Geometry: final body of the model. Coordinates: model frame, mm. A direction names the side the tool comes from. Give positions to 0.01 mm unless a question says otherwise; leave off trailing zeros. Order: outer loops, then holes, each group sorted by start corner. A loop starts at its lowest first (then second) coordinate and runs counter-clockwise, first axis right, second up. Notation, with made-up numbers: (86, 43.5) -> (114, 43.5) arc R22 ccw to (114, 68.5) -> close; hole circle Ø5 at (20.25, -31). An arc over 180 degrees is marked (long way). One line per item, written item: value. Start each with the question number.
```python
from build123d import *
from build123d.topology import SkipClean

# Parameters (mm, degrees)
BOSS_EXTRUDE1_DEPTH = 21
SKETCH2_R           = 12
CUT_EXTRUDE1_DEPTH  = 21
SKETCH3_R           = 26
CUT_EXTRUDE2_DEPTH  = 273.603191471
SKETCH5_R           = 31.5
SKETCH5_R_2         = 26
BOSS_EXTRUDE2_DEPTH = 35
SKETCH4_R           = 5
BOSS_EXTRUDE3_DEPTH = 7
CUT_EXTRUDE3_DEPTH  = 20
CUT_EXTRUDE5_REACH  = 280.977
CUT_EXTRUDE6_REACH  = 280.977
CUT_EXTRUDE7_START  = -2.5
CUT_EXTRUDE7_DEPTH  = 274.030851267


with BuildPart() as part:
    # Sketch1 → Boss-Extrude1 (new, symmetric)
    with BuildSketch(Plane(origin=(0, 0, 0), x_dir=(1, 0, 0), z_dir=(0, 1, 0))):
        with BuildLine():
            Line((60.430871603, 12.898377286), (220, 8.719912605))
            ThreePointArc((220, 8.719912605), (230.604685788, 10.075596562), (240.30539773, 14.569306326))
            ThreePointArc((240.30539773, 14.569306326), (267.5, 0), (240.30539773, -14.569306326))
            ThreePointArc((240.30539773, -14.569306326), (230.604685788, -10.075596562), (220, -8.719912605))
            Line((220, -8.719912605), (60.430871603, -12.898377286))
            ThreePointArc((60.430871603, -12.898377286), (37.890504435, -16.634432055), (17.222812986, -26.374698346))
            ThreePointArc((17.222812986, -26.374698346), (-31.5, 0), (17.222812986, 26.374698346))
            ThreePointArc((17.222812986, 26.374698346), (37.890504435, 16.634432055), (60.430871603, 12.898377286))
        make_face()
    extrude(amount=BOSS_EXTRUDE1_DEPTH, both=True)

    # Sketch2 → Cut-Extrude1 (cut, symmetric)
    with BuildSketch(Plane(origin=(0, 0, 0), x_dir=(1, 0, 0), z_dir=(0, 1, 0))):
        with Locations(Location((250, 0, 0), (0, 0, 270))):
            Circle(SKETCH2_R)
    extrude(amount=CUT_EXTRUDE1_DEPTH, both=True, mode=Mode.SUBTRACT)

    # Sketch3 → Cut-Extrude2 (cut, through all)
    with BuildSketch(Plane.XZ.offset(21)):
        with Locations(Location((0, 0, 0), (0, 0, 270))):
            Circle(SKETCH3_R)
    extrude(amount=-CUT_EXTRUDE2_DEPTH, mode=Mode.SUBTRACT)

    # Sketch5 → Boss-Extrude2 (add, symmetric)
    with SkipClean():  # the faces are left unmerged after this step: merging them gives an invalid solid
        with BuildSketch(Plane(origin=(0, 0, 0), x_dir=(1, 0, 0), z_dir=(0, 1, 0))):
            with Locations(Location((0, 0, 0), (0, 0, 270))):
                Circle(SKETCH5_R)
            with Locations(Location((0, 0, 0), (0, 0, 90))):
                Circle(SKETCH5_R_2, mode=Mode.SUBTRACT)
        extrude(amount=BOSS_EXTRUDE2_DEPTH, both=True)

    # Sketch4 → Boss-Extrude3 (add)
    with BuildSketch(Plane.XZ.offset(21)):
        with BuildLine():
            Line((87.482015231, 12.190018161), (87.482015231, -12.190018161))
            ThreePointArc((87.482015231, -12.190018161), (51.997088566, -22.622612499), (26.373739078, -49.29587638))
            ThreePointArc((26.373739078, -49.29587638), (17.709961948, -55.714405462), (7.181946677, -53.386435492))
            ThreePointArc((7.181946677, -53.386435492), (-14.855989459, -42.122318837), (-39.406288617, -38.986435492))
            ThreePointArc((-39.406288617, -38.986435492), (-50.326951915, -33.896458963), (-52.376901133, -22.023529412))
            ThreePointArc((-52.376901133, -22.023529412), (-48.925892025, 0), (-52.376901133, 22.023529412))
            ThreePointArc((-52.376901133, 22.023529412), (-50.326951915, 33.896458963), (-39.406288617, 38.986435492))
            ThreePointArc((-39.406288617, 38.986435492), (-14.855989459, 42.122318837), (7.181946677, 53.386435492))
            ThreePointArc((7.181946677, 53.386435492), (17.709961948, 55.714405462), (26.373739078, 49.29587638))
            ThreePointArc((26.373739078, 49.29587638), (51.997088566, 22.622612499), (87.482015231, 12.190018161))
        make_face()
        with Locations(Location((15, 43, 0), (0, 0, 270))):
            Circle(SKETCH4_R, mode=Mode.SUBTRACT)
        with Locations(Location((-40, 26, 0), (0, 0, 270))):
            Circle(SKETCH4_R, mode=Mode.SUBTRACT)
        with Locations(Location((15, -43, 0), (0, 0, 90))):
            Circle(SKETCH4_R, mode=Mode.SUBTRACT)
        with Locations(Location((-40, -26, 0), (0, 0, 90))):
            Circle(SKETCH4_R, mode=Mode.SUBTRACT)
    boss_extrude3 = extrude(amount=-BOSS_EXTRUDE3_DEPTH)

    # Mirror1: Boss-Extrude3 across plane
    add(boss_extrude3.mirror(Plane.ZX))

    # Sketch6 → Cut-Extrude3 (cut, symmetric)
    with BuildSketch(Plane.XY):
        with BuildLine():
            Line((123.875759549, 11.370189358), (232.5, 9))
            Line((232.5, 9), (232.5, 21))
            Line((232.5, 21), (88, 21))
            ThreePointArc((88, 21), (105.356268471, 14.018307807), (123.875759549, 11.370189358))
        make_face()
    cut_extrude3 = extrude(amount=CUT_EXTRUDE3_DEPTH, both=True, mode=Mode.SUBTRACT)

    # Mirror2: Cut-Extrude3 across plane
    add(cut_extrude3.mirror(Plane.ZX), mode=Mode.SUBTRACT)

    # Cut-Extrude5: up to this face of the body (flat: up to its plane)
    cut_extrude5_end = Plane(part.part.faces().sort_by_distance((176.036341328, 10.232041415, 0))[0])
    # Sketch7 → Cut-Extrude5 (cut, up to the picked face)
    with BuildSketch(Plane(origin=(0, 21, 0), x_dir=(1, 0, 0), z_dir=(0, 1, 0)), mode=Mode.PRIVATE) as cut_extrude5_sk1:
        with BuildLine():
            Line((232.5, 10.680424072), (232.5, 0))
            ThreePointArc((232.5, 0), (234.574282193, 8.264213825), (240.30539773, 14.569306326))
            ThreePointArc((240.30539773, 14.569306326), (236.524290746, 12.380817442), (232.5, 10.680424072))
        make_face()
    cut_extrude5_tool1 = split(extrude(cut_extrude5_sk1.sketch, amount=-CUT_EXTRUDE5_REACH, mode=Mode.PRIVATE), bisect_by=cut_extrude5_end, keep=Keep.BOTH, mode=Mode.PRIVATE)
    cut_extrude5 = cut_extrude5_tool1.solids().sort_by(Axis((234.203382, 21, -9.039339), (0, -1, 0)))[0]
    add(cut_extrude5, mode=Mode.SUBTRACT)

    # Mirror10: Cut-Extrude5 across plane
    with SkipClean():  # the faces are left unmerged after this step: merging them gives an invalid solid
        add(cut_extrude5.mirror(Plane.XY), mode=Mode.SUBTRACT)

    # Cut-Extrude6: up to this face of the body (flat: up to its plane)
    cut_extrude6_end = Plane(part.part.faces().sort_by_distance((176.036341328, -10.232041415, 0))[0])
    # Sketch9 → Cut-Extrude6 (cut, up to the picked face)
    with BuildSketch(Plane.XZ.offset(21), mode=Mode.PRIVATE) as cut_extrude6_sk1:
        with BuildLine():
            Line((232.5, 10.680424072), (232.5, 0))
            ThreePointArc((232.5, 0), (234.574282193, 8.264213825), (240.30539773, 14.569306326))
            ThreePointArc((240.30539773, 14.569306326), (236.524290746, 12.380817442), (232.5, 10.680424072))
        make_face()
    cut_extrude6_tool1 = split(extrude(cut_extrude6_sk1.sketch, amount=-CUT_EXTRUDE6_REACH, mode=Mode.PRIVATE), bisect_by=cut_extrude6_end, keep=Keep.BOTH, mode=Mode.PRIVATE)
    # Sketch9 → Cut-Extrude6 (cut, up to the picked face)
    with BuildSketch(Plane.XZ.offset(21), mode=Mode.PRIVATE) as cut_extrude6_sk2:
        with BuildLine():
            Line((232.5, 0), (232.5, -10.680424072))
            ThreePointArc((232.5, -10.680424072), (236.524290746, -12.380817442), (240.30539773, -14.569306326))
            ThreePointArc((240.30539773, -14.569306326), (234.574282193, -8.264213825), (232.5, 0))
        make_face()
    cut_extrude6_tool2 = split(extrude(cut_extrude6_sk2.sketch, amount=-CUT_EXTRUDE6_REACH, mode=Mode.PRIVATE), bisect_by=cut_extrude6_end, keep=Keep.BOTH, mode=Mode.PRIVATE)
    add(cut_extrude6_tool1.solids().sort_by(Axis((234.203382, -21, 9.039339), (0, 1, 0)))[0], mode=Mode.SUBTRACT)
    add(cut_extrude6_tool2.solids().sort_by(Axis((234.203382, -21, -9.039339), (0, 1, 0)))[0], mode=Mode.SUBTRACT)

    # Sketch10 → Cut-Extrude7 (cut, through all)
    with SkipClean():  # the faces are left unmerged after this step: merging them gives an invalid solid
        with BuildSketch(Plane(origin=(0, 0, 0), x_dir=(1, 0, 0), z_dir=(0, 1, 0)).offset(CUT_EXTRUDE7_START)):
            with BuildLine():
                Line((220, -6), (70, -6))
                ThreePointArc((70, -6), (64, 0), (70, 6))
                Line((70, 6), (220, 6))
                ThreePointArc((220, 6), (226, 0), (220, -6))
            make_face()
        cut_extrude7 = extrude(amount=-CUT_EXTRUDE7_DEPTH, mode=Mode.SUBTRACT)

    # Mirror11: Cut-Extrude7 across plane
    with SkipClean():  # the faces are left unmerged after this step: merging them gives an invalid solid
        add(cut_extrude7.mirror(Plane.ZX), mode=Mode.SUBTRACT)


solid = part.part
```
1. Cut plane B-B, the plane x = 250. Return loops of the section in (y, z).
2. Cut plane A-A, the plane y = -17. Return loops of the section in (x, z).
3. Draft query along X for faces 5 (the flat face through (0, 21, 0)), 6 (the cylindrical face through (-31.486, 0.196, 0.948)), 7 (the flat face through (26, -35, 5)). Return one class per face: pulls with the +X half, pulls with the -X half, needs draft (parallel to the pull), parting line crosses it, or undercut.
4. Access query for faces 1 (the cylindrical face through (105.103, 14.087, -9.045)), 2 (the flat face through (34, -21, -1)), 3 (the cylindrical face through (51.55, 17.549, 22.896)), 4 (the flat face through (34, 21, -1)). Directions: +Z, -Z, +X, -X, +Y, -Y. A direction counts if a zero-diameter tool reaches every point of the face in a straight line with its end or side. Return the directions, or none.
5. Pin query (flat end, axial travel): P1, Ø9, axis at x = 125, y = -14.5, coming from the +Z side; P2, Ø12, axis at x = 151.5, y = -16.5, coming from the -Z side; P3, Ø15, axis at x = 161.5, y = 15, coming from the -Z side. Return the tip coordinate at first contact, or that it passes through.
6. Cut plane C-C, the plane z = 43. Return loops of the section in (x, y).
7. Material intervals for L1, parallel to Z at x = 0, y = -32; L2, parallel to X at y = 11, z = 1, sorted ascending. Write a range as [from, to].
8. Cut plane D-D, the plane x = 183. Return loops of the section in (y, z), then the cut area to 3 significant figures.
Answers follow:
1. outline: (-21, -17.5) -> (21, -17.5) -> (21, -12) -> (-21, -12) -> close; (-21, 12) -> (21, 12) -> (21, 17.5) -> (-21, 17.5) -> close
2. outline: (-52.38, -22.02) arc R13 ccw to (-39.41, -38.99) arc R72 cw to (7.18, -53.39) arc R13 ccw to (26.37, -49.3) arc R72 cw to (87.48, -12.19) -> (96.44, -11.96) -> (96.44, -6) -> (70, -6) arc R6 cw to (70, 6) -> (96.44, 6) -> (96.44, 11.96) -> (87.48, 12.19) arc R72 cw to (26.37, 49.3) arc R13 ccw to (7.18, 53.39) arc R72 cw to (-39.41, 38.99) arc R13 ccw to (-52.38, 22.02) arc R72 cw to start; circle Ø35 at (250, 0); hole circle Ø10 at (-40, -26); hole circle Ø10 at (-40, 26); hole circle Ø10 at (15, -43); hole circle Ø10 at (15, 43); hole circle Ø24 at (250, 0)
3. face 5: undercut
3. face 6: parting line crosses it
3. face 7: needs draft
4. face 1: +Z, -Z, +Y
4. face 2: -Y
4. face 3: +Z, +Y, -Y
4. face 4: +Y
5. P1: stops at z = 11.29
5. P2: stops at z = -10.56
5. P3: stops at z = -10.41
6. outline: (-12.2, -21) -> (10, -21) -> (10, -14) -> (-12.2, -14) -> close; (-12.2, 14) -> (10, 14) -> (10, 21) -> (-12.2, 21) -> close; (20, -21) -> (30.3, -21) -> (30.3, -14) -> (20, -14) -> close; (20, 14) -> (30.3, 14) -> (30.3, 21) -> (20, 21) -> close
7. L1: z = [-31.5, -26], [26, 31.5]
7. L2: x = [-31.48, -25.98], [25.98, 64.08], [232.53, 238.04], [261.96, 267.47]
8. outline: (-10.08, -9.69) -> (10.08, -9.69) -> (10.08, -6) -> (2.5, -6) -> (2.5, 6) -> (10.08, 6) -> (10.08, 9.69) -> (-10.08, 9.69) -> (-10.08, 6) -> (-2.5, 6) -> (-2.5, -6) -> (-10.08, -6) -> close
8. area: 209 mm²
